Here's the drawing with two shaded views (mm, measured from the low corner). I have some questions. A direction names the side the tool comes from. Round coordinates to 2 decimals unless told otherwise and drop trailing zeros. Order: outer loops, then holes, each group sorted by start corner. A loop starts at its lowest first (then second) coordinate and runs counter-clockwise, first axis right, second up.
Q1. If we section it at A-A (x = 28): Please give me the cut outline in (y, z), plus the area to 3 significant figures.
Q2. If I drill on line 1 (X direction, y = 31, z = 26); line 2 (X direction, y = 3, z = 35); line 3 (Y direction, x = 17.5, z = 13), over which ranges is the centre line in solid material (lowest first)?
Q3. If we section it at D-D (y = 28): Please give me the cut outline in (x, z).
Q4. Will these pins go through, and if not, where does the flat tip stop? P1, Ø24, axis at y = 29.5, z = 27, coming from the +X side; P2, Ø10, axis at x = 16.5, y = 30, coming from the -Z side; P3, Ø10, axis at y = 20.5, z = 12.5, coming from the +X side (3 decimals).
Q5. If we section it at C-C (z = 18): Please give me the cut outline in (x, y), plus the area to 3 significant figures.
Q6. For the marked faces 1 and 2, which set-ups out of +Z, -Z, +X, -X, +Y, -Y let a thin tool reach every point of the face, with its end or its side?
Q7. If we section it at B-B (y = 34): Please give me the cut outline in (x, z).
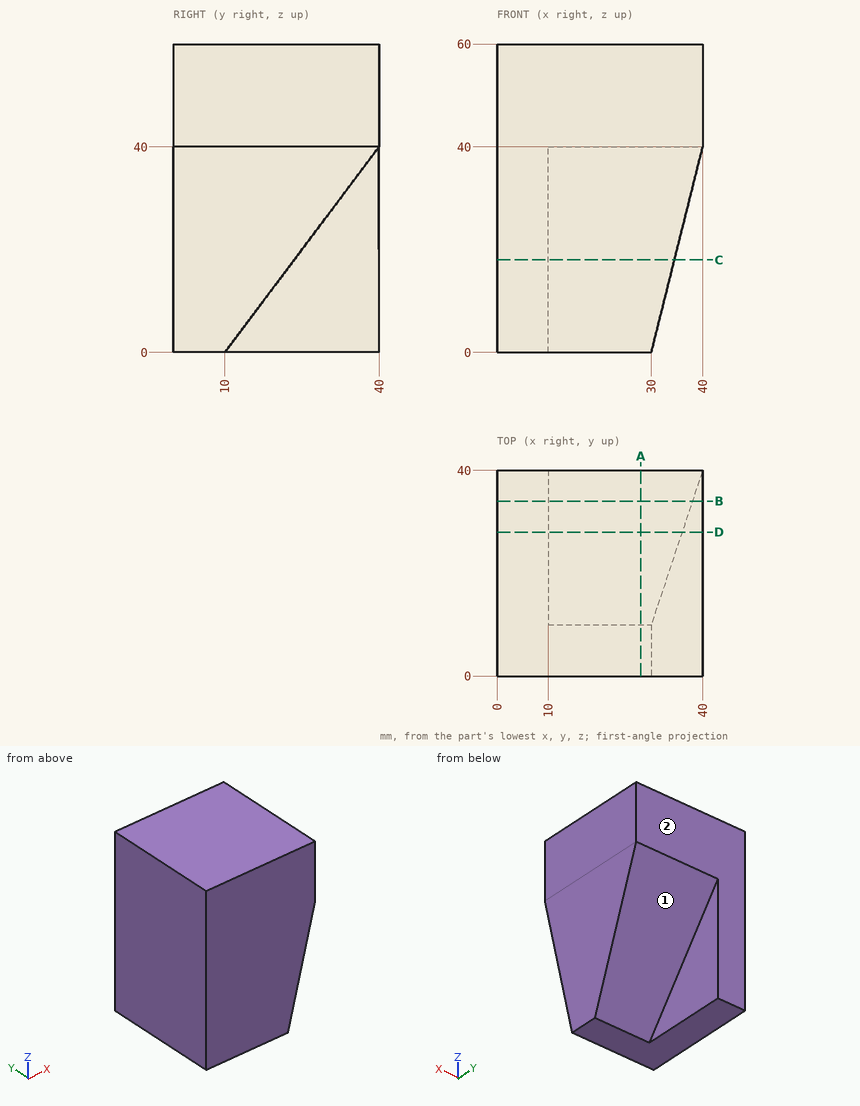
Solution:
1. outline: (0, 0) - (10, 0) - (40, 40) - (40, 60) - (0, 60) - close
1. area: 1,800 mm2
2. line 1: x = 0 to 10
2. line 2: x = 0 to 38.75
2. line 3: y = 0 to 19.75
3. outline: (0, 0) - (10, 0) - (10, 24) - (36, 24) - (40, 40) - (40, 60) - (0, 60) - close
4. P1: stops at x = 39.75
4. P2: stops at z = 20
4. P3: stops at x = 34.375
5. outline: (0, 0) - (34.5, 0) - (34.5, 23.5) - (10, 23.5) - (10, 40) - (0, 40) - close
5. area: 976 mm2
6. face 1: -Z, +X, +Y
6. face 2: +Z, -Z, +X, -X, +Y
7. outline: (0, 0) - (10, 0) - (10, 32) - (38, 32) - (40, 40) - (40, 60) - (0, 60) - close
